Input: part model. Units: mm. Frame: model coordinates. A direction names the side the tool comes from. Round coordinates to 2 decimals unless told otherwise and drop trailing zeros. Write each loop counter-clockwise with the first axis right and the second up, starting at its lowest first coordinate (ties: lowest second). Pieces come first, ordered by that corner, then holes. Notation, with made-up numbers: M -6,-9.5 L 7,-9.5 A8 ccw 7,2.5 Z; hole C -5.5,43.25 d10. An arc over 180 degrees is marked long. Answer as CSV lines item,"result". Start each with the question number.
```python
from build123d import *

# Parameters (mm, degrees)
F0_W      = 80
F0_H      = 29
F1_DEPTH  = 3
F2_W      = 80
F2_H      = 3
F3_DEPTH  = 10
F4_R      = 5
F6_D      = 3
F7_W      = 2
F7_H      = 5
F8_ANGLE  = 90
F9_W      = 2
F9_H      = 5
F10_ANGLE = 90


with BuildPart() as f1:
    # F0 (on Top) → F1 (new body)
    with BuildSketch(Plane.XY):
        Rectangle(F0_W, F0_H)
    extrude(amount=F1_DEPTH)

    # F2 (on face) → F3 (join)
    with BuildSketch(Plane.XY.offset(3)):
        with Locations((0, 3)):
            Rectangle(F2_W, F2_H)
        with Locations((0, -3)):
            Rectangle(F2_W, F2_H)
    extrude(amount=F3_DEPTH)

    # F4
    f4_edges = [f1.edges().sort_by_distance(p)[0] for p in [
        (40, 14.5, 1.5),
        (40, -14.5, 1.5),
        (-40, 14.5, 1.5),
        (-40, -14.5, 1.5),
        (40, 3, 13),
        (40, -3, 13),
        (-40, 3, 13),
        (-40, -3, 13),
    ]]
    fillet(f4_edges, radius=F4_R)

    # F6 (through all)
    with Locations(Plane.XY.offset(3)):
        with Locations((-30, 9.5), (-30, -9.5), (30, -9.5), (30, 9.5)):
            Hole(F6_D / 2)

    # F7 (on face) → F8 (revolve)
    with BuildSketch(Plane(origin=(0, 4.5, 0), x_dir=(-1, 0, 0), z_dir=(0, 1, 0))):
        with Locations((-21, 5.5)):
            Rectangle(F7_W, F7_H)
        with Locations((21, 5.5)):
            Rectangle(F7_W, F7_H)
    revolve(axis=Axis((21, 4.5, 3), (-1, 0, 0)), revolution_arc=F8_ANGLE)

    # F9 (on face) → F10 (revolve)
    with BuildSketch(Plane.XZ.offset(4.5)):
        with Locations((-21.000002, 5.5)):
            Rectangle(F9_W, F9_H)
        with Locations((21.000002, 5.5)):
            Rectangle(F9_W, F9_H)
    revolve(axis=Axis((-21.000002, -4.5, 3), (1, 0, 0)), revolution_arc=F10_ANGLE)


solid = f1.part
```
Item 1: Access query for faces 4 (the face through (-1, 10, 3)), 5 (the face through (-22, 6, 5)), 6 (the face through (22, 6, 5)). Directions: +Z, -Z, +X, -X, +Y, -Y. A direction counts if a zero-diameter tool reaches every point of the face in a straight line with its end or side. Return the directions, or none.
Item 2: Line query: line 1 (Y direction, x = 30, z = 1.5); line 2 (Y direction, x = 36.5, z = 4); line 3 (Z direction, x = -14, y = -7.5). Output: solid intervals per line, ascending. Write a range as [from, to].
Item 3: Cut plane A-A, the plane x = 30. Return loops of the section in (y, z), plus the area to 3 significant figures.
Item 4: Cut plane D-D, the plane x = -16. Return loops of the section in (y, z).
Item 5: Cut plane B-B, the plane z = 1. Return loops of the section in (x, y), plus the area to 3 significant figures.
Item 6: Draft query along Y for faces 1 (the face through (21.01, -8, 6.57)), 2 (the face through (-21.01, 8, 6.57)), 3 (the face through (31.5, -9.43, 1.48)). Return one class per face: +Y half, -Y half, draft (parallel to the pull), parting line (faces both ways), or undercut.
Item 7: Pin query (flat end, axial travel): pin 1 Ø3 at (x, z) = (14.5, 7) entering from -Y; pin 2 Ø2.5 at (y, z) = (6, 4.5) entering from -X; pin 3 Ø3.5 at (x, y) = (30, 9.5) entering from +Z. Return the tip coordinate at first contact, or that it passes through.
Item 8: Cut plane C-C, the plane z = 9.75. Return loops of the section in (x, y), plus the area to 3 significant figures.
Results list:
1,face 4,"+Z, +Y"
1,face 5,"+Z, -X, +Y"
1,face 6,"+Z, +X, +Y"
2,line 1,"[-14.5, -11], [-8, 8], [11, 14.5]"
2,line 2,"[-4.5, -1.5], [1.5, 4.5]"
2,line 3,"[0, 3]"
3,outline,"M -14.5,0 L -11,0 L -11,3 L -14.5,3 Z; M -8,0 L 8,0 L 8,3 L 4.5,3 L 4.5,13 L 1.5,13 L 1.5,3 L -1.5,3 L -1.5,13 L -4.5,13 L -4.5,3 L -8,3 Z; M 11,0 L 14.5,0 L 14.5,3 L 11,3 Z"
3,area,"129 mm²"
4,outline,"M -14.5,0 L 14.5,0 L 14.5,3 L 4.5,3 L 4.5,13 L 1.5,13 L 1.5,3 L -1.5,3 L -1.5,13 L -4.5,13 L -4.5,3 L -14.5,3 Z"
5,outline,"M -40,-9.5 A5 ccw -35,-14.5 L 35,-14.5 A5 ccw 40,-9.5 L 40,9.5 A5 ccw 35,14.5 L -35,14.5 A5 ccw -40,9.5 Z; hole C -30,-9.5 d3; hole C -30,9.5 d3; hole C 30,-9.5 d3; hole C 30,9.5 d3"
5,area,"2,270 mm²"
6,face 1,"-Y half"
6,face 2,"+Y half"
6,face 3,"undercut"
7,pin 1,"y = -4.5"
7,pin 2,"x = -22"
7,pin 3,"z = 3"
8,outline,"M -39.68,-4.5 L 39.68,-4.5 L 39.68,-1.5 L -39.68,-1.5 Z; M -39.68,1.5 L 39.68,1.5 L 39.68,4.5 L -39.68,4.5 Z"
8,area,"476 mm²"
